Work out the finished part from the listing and answer in its coordinate system (mm). A direction names the side the tool comes from. Round coordinates to 2 decimals unless told otherwise and drop trailing zeros. Order: outer loops, then holes, each group sorted by start corner. A loop starts at its lowest first (then second) coordinate and runs counter-clockwise, first axis right, second up. Notation, with made-up numbers: (13.25, 31.25) - (48.25, 31.25) arc R21 ccw to (48.25, 50.25) - close; hole circle Ø4 at (1, 41). An arc over 180 degrees is marked (long way). Put each result on its own line as item: value.
```python
from build123d import *

# Parameters (mm, degrees)
EXTRUDE004_DEPTH = 2.45
EXTRUDE_DEPTH    = 4.5
EXTRUDE006_DEPTH = 30
EXTRUDE005_DEPTH = 3
PAD_DEPTH        = 5
PAD_DEPTH_BACK   = -5
SKETCH015_R      = 1.8
POCKET_DEPTH     = 14
SKETCH017_R      = 4
PAD001_DEPTH     = 10


with BuildPart() as extrude004:
    # Sketch008 (on Face9 of Extrude) → Extrude004 (new body)
    with BuildSketch(Plane(origin=(0, 0, 4.5), x_dir=(0, 1, 0), z_dir=(0, 0, 1))):
        with BuildLine():
            Line((0, 19), (2.9, 19))
            Line((2.9, 19), (2.9, 15.682663))
            Line((4.4, 4.079216), (2.9, 15.682663))
            ThreePointArc((6, 0), (5.585696, 2.19089), (4.4, 4.079216))
            Line((0, 0), (6, 0))
            Line((0, 0), (0, 19))
        make_face()
    extrude(amount=-EXTRUDE004_DEPTH)


with BuildPart() as fusion003:
    # Part__Mirroring002: instance of Extrude004
    add(extrude004.part.mirror(Plane(origin=(0, 0, 0), x_dir=(0, -1, 0), z_dir=(1, 0, 0))))

    # Fusion003: union Extrude004
    add(extrude004.part)


with BuildPart() as cut:
    # Sketch001 → Extrude (new body)
    with BuildSketch(Plane.XY):
        with BuildLine():
            ThreePointArc((-200, 5.572639), (-196.759552, 8.020606), (-195.948707, 12))
            Line((-195.948707, 12), (-49.447849, 12))
            add(Edge.make_bspline(
                [(4.051293, 7), (-44.340996, 6.588548), (-49.447849, 12)],
                knots=[0, 0, 0, 1, 1, 1], degree=2))
            ThreePointArc((4.051293, 7), (9.785764, 5.613765), (11.6, 0))
            Line((11.6, 0), (1.6, 0))
            ThreePointArc((1.6, 0), (0, 1.6), (-1.6, 0))
            Line((-1.6, 0), (-90.499023, 0))
            Line((-90.499023, 0), (-197, 0))
            ThreePointArc((-197, 0), (-200, 3), (-203, 0))
            Line((-203, 0), (-205.572639, 0))
            ThreePointArc((-205.572639, 0), (-203.940451, 3.940451), (-200, 5.572639))
        make_face()
    extrude(amount=EXTRUDE_DEPTH)

    # Cut: cut Fusion003
    add(fusion003.part, mode=Mode.SUBTRACT)


with BuildPart() as part_mirroring:
    # Part__Mirroring: instance of Cut
    add(cut.part.mirror(Plane(origin=(0, 0, 0), x_dir=(1, 0, 0), z_dir=(0, 1, 0))))


with BuildPart() as fusion:
    # Fusion base: copy of Cut
    add(cut.part)

    # Fusion: union Part__Mirroring
    add(part_mirroring.part)


with BuildPart() as extrude006:
    # Sketch013 → Extrude006 (new body, symmetric)
    with BuildSketch(Plane.XZ):
        Polygon((-190, 5), (-22.11842, 7), (-190, 7), align=None)
    extrude(amount=EXTRUDE006_DEPTH, both=True)


with BuildPart() as body:
    # Sketch012 → Extrude005 (new body)
    with BuildSketch(Plane.XY.offset(4)):
        with BuildLine():
            Line((-185.354797, 11.026761), (-22.840828, 5.142419))
            ThreePointArc((-22.840828, -5.142419), (-20.938647, 0), (-22.840828, 5.142419))
            Line((-22.840828, -5.142419), (-185.354797, -11.026761))
            Line((-185.354797, -11.026761), (-185.354797, -5.026761))
            Line((-185.354797, -5.026761), (-28.840828, 0))
            Line((-28.840828, 0), (-185.354797, 5.026761))
            Line((-185.354797, 5.026761), (-185.354797, 11.026761))
        make_face()
    extrude(amount=EXTRUDE005_DEPTH)

    # Cut001: cut Extrude006
    add(extrude006.part, mode=Mode.SUBTRACT)

    # Fusion004: union Fusion
    add(fusion.part)

    # Sketch → Pad (new body, two sides)
    with BuildSketch(Plane.XZ) as pad_sk:
        with BuildLine():
            ThreePointArc((-15, 4.5), (-19, 8.5), (-23, 4.5))
            Line((-23, 4.5), (-15, 4.5))
        make_face()
    extrude(amount=-PAD_DEPTH)
    extrude(pad_sk.sketch, amount=-PAD_DEPTH_BACK)

    # Sketch015 → Pocket (cut, symmetric)
    with BuildSketch(Plane.XY.offset(4)):
        with Locations((-10, 0)):
            Circle(SKETCH015_R)
    extrude(amount=POCKET_DEPTH, both=True, mode=Mode.SUBTRACT)

    # Sketch017 (on Face7 of Pocket) → Pad001 (join)
    with BuildSketch(Plane(origin=(-113.60842, 0, 4.5), x_dir=(0, 1, 0), z_dir=(0, 0, 1))):
        with Locations((0, 67.406453)):
            Circle(SKETCH017_R)
    extrude(amount=PAD001_DEPTH)


solid = body.part
```
1) Given pin 1 Ø3 at (x, y) = (-17.5, -0.5) entering from -Z; pin 2 Ø0.6 at (y, z) = (-9.5, 5) entering from -X; pin 3 Ø6.5 at (x, y) = (-5.5, -2.5) entering from +Z; pin 4 Ø1.2 at (x, z) = (-16.5, 4) entering from +Y, each flat-ended and moving along its own axis, determine where each tip first touches the part or whether it passes through.
Findings below:
pin 1: stops at z = 0
pin 2: stops at x = -185.35
pin 3: stops at z = 4.5
pin 4: stops at y = 7.15
2) For faces 4 (the flat face through (-17, 0, 4.5)), 5 (the cylindrical face through (-184.98, -0.52, 9.43)), 6 (the flat face through (-19, -5, 6)), determine the directions among +Z, -Z, +X, -X, +Y, -Y from which every point of the face is accessible in a straight line to the end or side of a thin tool.
Findings below:
face 4: +X
face 5: +Z
face 6: +Z, +X, -Y
3) A cutting plane is placed at B-B on z = 11. Write down the section's boundary in (x, y), then the cut area to 3 significant figures.
Findings below:
outline: circle Ø8 at (-181.01, 0)
area: 50.3 mm2
4) For a pull along X with two mould halves and no side action, classify faces 1 (the flat face through (-87.178, 7.472, 5.451)), 2 (the flat face through (-120, 0, 4.5)), 3 (the flat face through (-181, 0, 14.5)) as pulls with the +X half, pulls with the -X half, needs draft (parallel to the pull), parting line crosses it, or undercut.
Findings below:
face 1: pulls with the +X half
face 2: undercut
face 3: needs draft
5) Straight lines are drawn through the part: L1, parallel to Z at x = -191, y = -9.25; L2, parallel to X at y = 2.75, z = 4.25; L3, parallel to Y at x = -10, z = 1. For each, find the intervals that lie inside material, in ascending order. Write a range as from..to.
Findings below:
L1: z = 0..4.5
L2: x = -204.85..-201.2, -198.8..-19
L3: y = -7.01..-1.8, 1.8..7.01
6) A cutting plane is placed at C-C on x = -66.5. Write down the section's boundary in (y, z).
Findings below:
outline: (-12, 0) - (12, 0) - (12, 4.5) - (6.72, 4.5) - (6.72, 6.47) - (1.21, 6.47) - (1.21, 4.5) - (-1.21, 4.5) - (-1.21, 6.47) - (-6.72, 6.47) - (-6.72, 4.5) - (-12, 4.5) - close
7) A cutting plane is placed at A-A on x = -151. Write down the section's boundary in (y, z), then the cut area to 3 significant figures.
Findings below:
outline: (-12, 0) - (12, 0) - (12, 4.5) - (9.78, 4.5) - (9.78, 5.46) - (3.92, 5.46) - (3.92, 4.5) - (-3.92, 4.5) - (-3.92, 5.46) - (-9.78, 5.46) - (-9.78, 4.5) - (-12, 4.5) - close
area: 119 mm2
